```python
from build123d import *

# Parameters (mm, degrees)
ESQUISSE1_W            = 30
ESQUISSE1_H            = 30
BASE_PLATE_DEPTH       = 2
SKETCH_PERFORATIONS_R  = 0.6
CUT_PERFORATIONS_DEPTH = 10


with BuildPart() as part:
    # Esquisse1 → Base_Plate (new body)
    with BuildSketch(Plane.XY):
        Rectangle(ESQUISSE1_W, ESQUISSE1_H)
    extrude(amount=BASE_PLATE_DEPTH)

    # Sketch_Perforations → Cut_Perforations (cut)
    with BuildSketch(Plane.XY.offset(2)):
        with Locations((-4.14, -10.64)):
            Circle(SKETCH_PERFORATIONS_R)
        with Locations((-4.14, -8.27)):
            Circle(SKETCH_PERFORATIONS_R)
        with Locations((-4.14, -5.91)):
            Circle(SKETCH_PERFORATIONS_R)
        with Locations((-4.14, -3.55)):
            Circle(SKETCH_PERFORATIONS_R)
        with Locations((-4.14, -1.18)):
            Circle(SKETCH_PERFORATIONS_R)
        with Locations((-4.14, 1.18)):
            Circle(SKETCH_PERFORATIONS_R)
        with Locations((-4.14, 3.55)):
            Circle(SKETCH_PERFORATIONS_R)
        with Locations((-4.14, 5.91)):
            Circle(SKETCH_PERFORATIONS_R)
        with Locations((-4.14, 8.27)):
            Circle(SKETCH_PERFORATIONS_R)
        with Locations((-4.14, 10.64)):
            Circle(SKETCH_PERFORATIONS_R)
        with Locations((-2.07, -10.64)):
            Circle(SKETCH_PERFORATIONS_R)
        with Locations((-2.07, -8.27)):
            Circle(SKETCH_PERFORATIONS_R)
        with Locations((-2.07, -5.91)):
            Circle(SKETCH_PERFORATIONS_R)
        with Locations((-2.07, -3.55)):
            Circle(SKETCH_PERFORATIONS_R)
        with Locations((-2.07, -1.18)):
            Circle(SKETCH_PERFORATIONS_R)
        with Locations((-2.07, 1.18)):
            Circle(SKETCH_PERFORATIONS_R)
        with Locations((-2.07, 3.55)):
            Circle(SKETCH_PERFORATIONS_R)
        with Locations((-2.07, 5.91)):
            Circle(SKETCH_PERFORATIONS_R)
        with Locations((-2.07, 8.27)):
            Circle(SKETCH_PERFORATIONS_R)
        with Locations((-2.07, 10.64)):
            Circle(SKETCH_PERFORATIONS_R)
        with Locations((0, -10.64)):
            Circle(SKETCH_PERFORATIONS_R)
        with Locations((0, -8.27)):
            Circle(SKETCH_PERFORATIONS_R)
        with Locations((0, -5.91)):
            Circle(SKETCH_PERFORATIONS_R)
        with Locations((0, -3.55)):
            Circle(SKETCH_PERFORATIONS_R)
        with Locations((0, -1.18)):
            Circle(SKETCH_PERFORATIONS_R)
        with Locations((0, 1.18)):
            Circle(SKETCH_PERFORATIONS_R)
        with Locations((0, 3.55)):
            Circle(SKETCH_PERFORATIONS_R)
        with Locations((0, 5.91)):
            Circle(SKETCH_PERFORATIONS_R)
        with Locations((0, 8.27)):
            Circle(SKETCH_PERFORATIONS_R)
        with Locations((0, 10.64)):
            Circle(SKETCH_PERFORATIONS_R)
        with Locations((2.07, -10.64)):
            Circle(SKETCH_PERFORATIONS_R)
        with Locations((2.07, -8.27)):
            Circle(SKETCH_PERFORATIONS_R)
        with Locations((2.07, -5.91)):
            Circle(SKETCH_PERFORATIONS_R)
        with Locations((2.07, -3.55)):
            Circle(SKETCH_PERFORATIONS_R)
        with Locations((2.07, -1.18)):
            Circle(SKETCH_PERFORATIONS_R)
        with Locations((2.07, 1.18)):
            Circle(SKETCH_PERFORATIONS_R)
        with Locations((2.07, 3.55)):
            Circle(SKETCH_PERFORATIONS_R)
        with Locations((2.07, 5.91)):
            Circle(SKETCH_PERFORATIONS_R)
        with Locations((2.07, 8.27)):
            Circle(SKETCH_PERFORATIONS_R)
        with Locations((2.07, 10.64)):
            Circle(SKETCH_PERFORATIONS_R)
        with Locations((4.14, -10.64)):
            Circle(SKETCH_PERFORATIONS_R)
        with Locations((4.14, -8.27)):
            Circle(SKETCH_PERFORATIONS_R)
        with Locations((4.14, -5.91)):
            Circle(SKETCH_PERFORATIONS_R)
        with Locations((4.14, -3.55)):
            Circle(SKETCH_PERFORATIONS_R)
        with Locations((4.14, -1.18)):
            Circle(SKETCH_PERFORATIONS_R)
        with Locations((4.14, 1.18)):
            Circle(SKETCH_PERFORATIONS_R)
        with Locations((4.14, 3.55)):
            Circle(SKETCH_PERFORATIONS_R)
        with Locations((4.14, 5.91)):
            Circle(SKETCH_PERFORATIONS_R)
        with Locations((4.14, 8.27)):
            Circle(SKETCH_PERFORATIONS_R)
        with Locations((4.14, 10.64)):
            Circle(SKETCH_PERFORATIONS_R)
    extrude(amount=-CUT_PERFORATIONS_DEPTH, mode=Mode.SUBTRACT)


solid = part.part
```
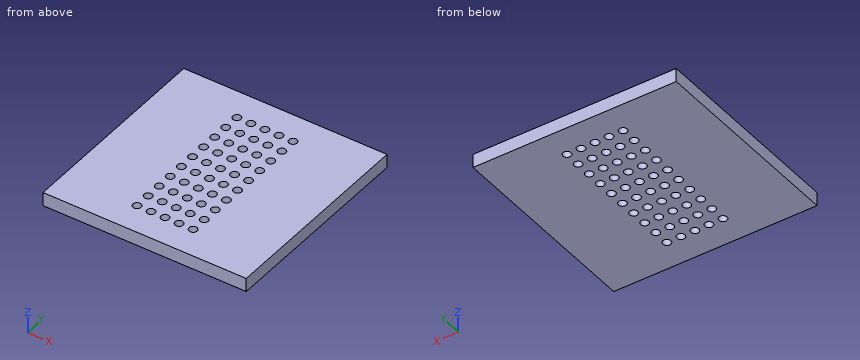
Verification items for the finished model (mm, model axes). Round coordinates to 2 decimals unless told otherwise and drop trailing zeros. Order: outer loops, then holes, each group sorted by start corner. A loop starts at its lowest first (then second) coordinate and runs counter-clockwise, first axis right, second up. Notation, with made-up numbers: (-11, -11) -> (29, -11) arc R36 ccw to (29, 26) -> close; hole circle Ø5 at (59, 9). An arc over 180 degrees is marked (long way). Put each result on its own line as item: value. Start each with the question number.
(1) Section check B-B (z = 0.85). State how many separate pieces and enclosed holes the cut face has, then the cut area to 3 significant figures.
(2) Depth check by flat-ended pin: pin 1 Ø0.7 at (x, y) = (-2.07, -1.18) entering from +Z. Enter the tip coordinate at first touch or a pass-through.
(3) Material ranges on line 1 along X through (y, z) = (-3.5, 1.2); line 2 along X through (y, z) = (10.5, 0.1), recorded low to high.
(4) Section check A-A (y = -1.18). Enter the section's corners in (x, z), then the cut area to 3 significant figures.
Completed:
1. separate pieces: 1
1. enclosed holes: 50
1. area: 843 mm2
2. pin 1: passes through
3. line 1: x = -15 to -4.74, -3.54 to -2.67, -1.47 to -0.6, 0.6 to 1.47, 2.67 to 3.54, 4.74 to 15
3. line 2: x = -15 to -4.72, -3.56 to -2.65, -1.49 to -0.58, 0.58 to 1.49, 2.65 to 3.56, 4.72 to 15
4. outline: (-15, 0) -> (-4.74, 0) -> (-4.74, 2) -> (-15, 2) -> close; (-3.54, 0) -> (-2.67, 0) -> (-2.67, 2) -> (-3.54, 2) -> close; (-1.47, 0) -> (-0.6, 0) -> (-0.6, 2) -> (-1.47, 2) -> close; (0.6, 0) -> (1.47, 0) -> (1.47, 2) -> (0.6, 2) -> close; (2.67, 0) -> (3.54, 0) -> (3.54, 2) -> (2.67, 2) -> close; (4.74, 0) -> (15, 0) -> (15, 2) -> (4.74, 2) -> close
4. area: 48.0 mm2
